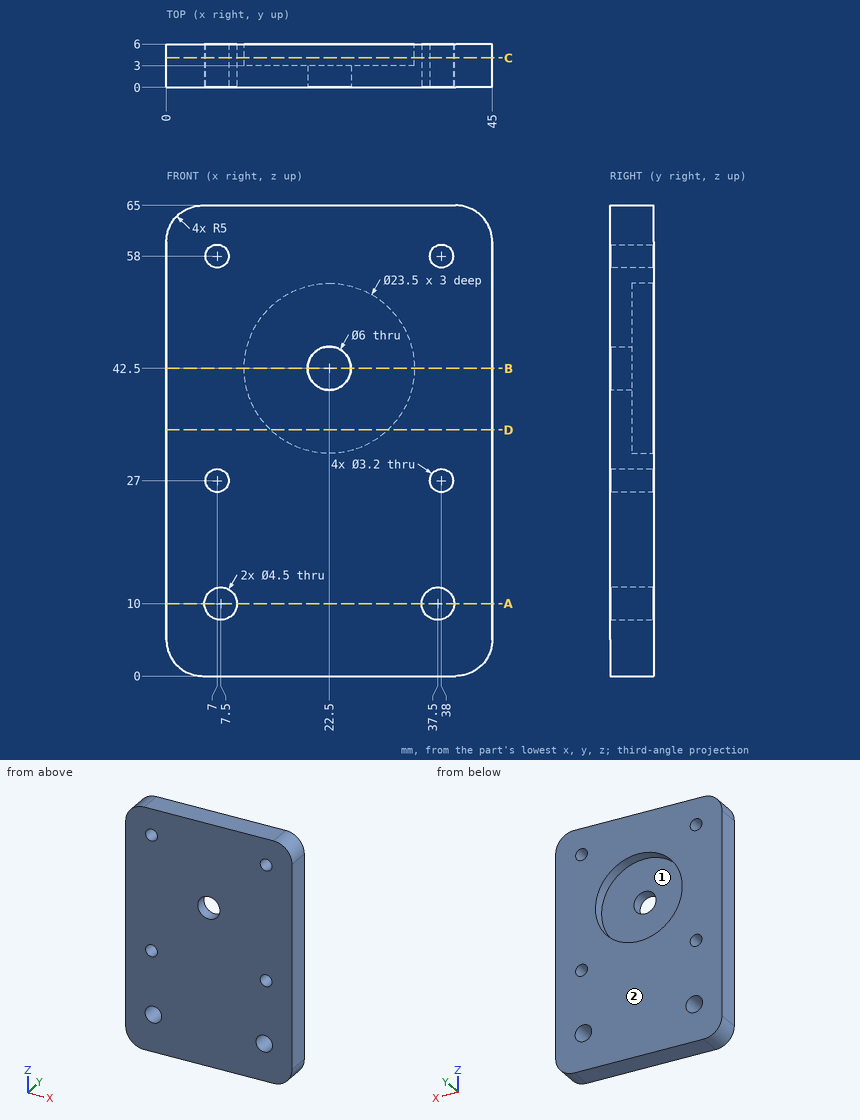
Design review of the part shown in the three views and the two pictorial views. Dimensions are in mm from the part's minimum x, y and z. Coordinates: 2 decimals unless noted, no trailing zeros. Order: outer loops, then holes, each group sorted by start corner. A loop starts at its lowest first (then second) coordinate and runs counter-clockwise, first axis right, second up.
1) Take a section at B-B, the plane z = 42.5. Give the boundary of the cut face in (x, y).
2) Wall thickness on line 1 along X through (y, z) = (4.5, 10); line 2 along X through (y, z) = (3.05, 26.5); line 3 along Z through (x, y) = (37.5, 3.65): over which ranges is each line inside the solid? List them lowest first.
3) Take a section at D-D, the plane z = 34. Give the boundary of the cut face in (x, y), and give its area (3 significant figures).
4) Take a section at A-A, the plane z = 10. Give the boundary of the cut face in (x, y).
5) Mouldability with a two-part tool opening along X and no side actions: class the marked faces 1 and 2 as +X half, -X half, draft (parallel to the pull), parting line (faces both ways), or undercut.
6) Take a section at C-C, the plane y = 4.1. Give the boundary of the cut face in (x, z), and give its area (3 significant figures).
7) Clearance check with flat-ended pins moving along their axes: pin 1 (3.5 mm diameter, centred on x = 37.5, z = 10, fed in from -Y); pin 2 (12 mm diameter, centred on x = 25.5, z = 43, fed in from +Y). State where each tip first meets the part, or that it passes through.
Returned:
1. outline: (0, 0) - (19.5, 0) - (19.5, 3) - (10.75, 3) - (10.75, 6) - (0, 6) - close; (25.5, 0) - (45, 0) - (45, 6) - (34.25, 6) - (34.25, 3) - (25.5, 3) - close
2. line 1: x = 0 to 5.25, 9.75 to 35.25, 39.75 to 45
2. line 2: x = 0 to 5.48, 8.52 to 36.48, 39.52 to 45
2. line 3: z = 0 to 7.75, 12.25 to 25.48, 28.52 to 56.48, 59.52 to 65
3. outline: (0, 0) - (45, 0) - (45, 6) - (30.61, 6) - (30.61, 3) - (14.39, 3) - (14.39, 6) - (0, 6) - close
3. area: 221 mm2
4. outline: (0, 0) - (5.25, 0) - (5.25, 6) - (0, 6) - close; (9.75, 0) - (35.25, 0) - (35.25, 6) - (9.75, 6) - close; (39.75, 0) - (45, 0) - (45, 6) - (39.75, 6) - close
5. face 1: undercut
5. face 2: draft
6. outline: (0, 5) arc R5 ccw to (5, 0) - (40, 0) arc R5 ccw to (45, 5) - (45, 60) arc R5 ccw to (40, 65) - (5, 65) arc R5 ccw to (0, 60) - close; hole circle Ø4.5 at (7.5, 10); hole circle Ø3.2 at (7, 27); hole circle Ø3.2 at (7, 58); hole circle Ø23.5 at (22.5, 42.5); hole circle Ø4.5 at (37.5, 10); hole circle Ø3.2 at (38, 27); hole circle Ø3.2 at (38, 58)
6. area: 2,410 mm2
7. pin 1: passes through
7. pin 2: stops at y = 3
